```python
from build123d import *

# Parameters (mm, degrees)
SKETCH1_W            = 43.18
SKETCH1_H            = 43.18
BOSS_EXTRUDE1_DEPTH  = 43.18
SKETCH2_R            = 5
BOSS_EXTRUDE2_DEPTH  = 25.4
SKETCH3_R            = 1.27
CUT_EXTRUDE1_DEPTH   = 43.18
LPATTERN1_COUNT      = 2
LPATTERN1_PITCH      = 35.9156
LPATTERN1_COUNT_DIR2 = 2
LPATTERN1_PITCH_DIR2 = 35.9156


with BuildPart() as part:
    # Sketch1 → Boss-Extrude1 (new body)
    with BuildSketch(Plane(origin=(0, 0, 0), x_dir=(1, 0, 0), z_dir=(0, 1, 0))):
        Rectangle(SKETCH1_W, SKETCH1_H)
    extrude(amount=BOSS_EXTRUDE1_DEPTH)

    # Sketch2 → Boss-Extrude2 (add)
    with BuildSketch(Plane(origin=(0, 43.18, 0), x_dir=(1, 0, 0), z_dir=(0, 1, 0))):
        Circle(SKETCH2_R)
    extrude(amount=BOSS_EXTRUDE2_DEPTH)

    # Sketch3 → Cut-Extrude1 (cut)
    with BuildSketch(Plane(origin=(0, 43.18, 0), x_dir=(1, 0, 0), z_dir=(0, 1, 0))):
        with Locations((-17.960512242, 17.960512242)):
            Circle(SKETCH3_R)
    cut_extrude1 = extrude(amount=-CUT_EXTRUDE1_DEPTH, mode=Mode.SUBTRACT)

    # LPattern1: Cut-Extrude1 2 × 2
    with Locations(*[(i * LPATTERN1_PITCH, 0, j * LPATTERN1_PITCH_DIR2) for i in range(LPATTERN1_COUNT) for j in range(LPATTERN1_COUNT_DIR2) if (i, j) != (0, 0)]):
        add(cut_extrude1, mode=Mode.SUBTRACT)


solid = part.part
```
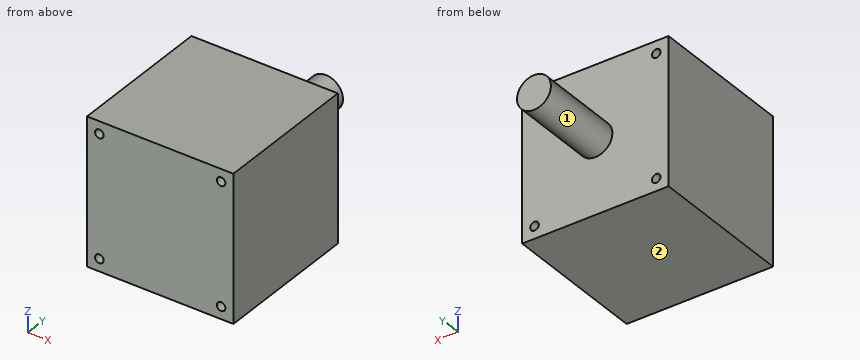
Input: part model. Units: mm. Frame: model coordinates. Face numbers are marked on the shaded views. A direction names the side the tool comes from. Give positions to 0.01 mm unless a question says otherwise; leave off trailing zeros. Order: outer loops, then holes, each group sorted by start corner. A loop starts at its lowest first (then second) coordinate and runs counter-clockwise, first axis right, second up. Notation, with made-up numbers: (43.25, -34) - (66.25, -34) arc R21 ccw to (66.25, -27) - close; hole circle Ø2 at (6.25, -8.5). An arc over 180 degrees is marked (long way). Put each result on its own line as item: value.
Item 1: Access query for the marked faces 1 and 2. Directions: +Z, -Z, +X, -X, +Y, -Y. A direction counts if a zero-diameter tool reaches every point of the face in a straight line with its end or side. Return the directions, or none.
Found:
face 1: +Y
face 2: -Z, +X, -X, +Y, -Y
Item 2: Contact query for flat-ended pins moving along their axis: pin 1 (1.5 mm diameter, centred on x = 17.96, z = 17.96, fed in from -Y); pin 2 (2 mm diameter, centred on x = 12, z = -3.5, fed in from +Y); pin 3 (10 mm diameter, centred on y = 57, z = 1.5, fed in from +X). Output: stop coordinate, or through.
Found:
pin 1: passes through
pin 2: stops at y = 43.18
pin 3: stops at x = 5
Item 3: Ray query, L1, parallel to Y at x = -12, z = 20; L2, parallel to X at y = 51, z = 1.5; L3, parallel to X at y = 57.5, z = 2.5. Return the intervals inside material, ascending. Write a range as from..to.
Found:
L1: y = 0..43.18
L2: x = -4.77..4.77
L3: x = -4.33..4.33
Item 4: Section query A-A, the plane x = 0. Return loops of the section in (y, z).
Found:
outline: (0, -21.59) - (43.18, -21.59) - (43.18, -5) - (68.58, -5) - (68.58, 5) - (43.18, 5) - (43.18, 21.59) - (0, 21.59) - close
Item 5: Section query D-D, the plane x = 12. Return loops of the section in (y, z).
Found:
outline: (0, -21.59) - (43.18, -21.59) - (43.18, 21.59) - (0, 21.59) - close
Item 6: Section query B-B, the plane z = 0. Return loops of the section in (x, y).
Found:
outline: (-21.59, 0) - (21.59, 0) - (21.59, 43.18) - (5, 43.18) - (5, 68.58) - (-5, 68.58) - (-5, 43.18) - (-21.59, 43.18) - close
Item 7: Section query C-C, the plane y = 47. Return loops of the section in (x, z), then the cut area to 3 significant figures.
Found:
outline: circle Ø10 at (0, 0)
area: 78.5 mm^2
